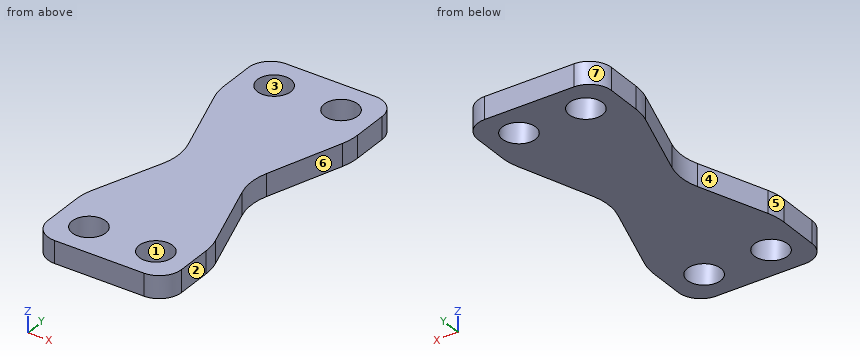
```python
from build123d import *

# Parameters (mm, degrees)
F0_R     = 1.5
F1_DEPTH = 2


with BuildPart() as f1:
    # F0 (on Top) → F1 (new body)
    with BuildSketch(Plane.XY):
        with BuildLine():
            ThreePointArc((-57.214044, -21.459296), (-56.628257, -22.87351), (-55.214044, -23.459296))
            Line((-55.214044, -23.459296), (-47.214044, -23.459296))
            ThreePointArc((-47.214044, -23.459296), (-45.79983, -22.87351), (-45.214044, -21.459296))
            Line((-45.214044, -21.459296), (-45.214044, -18.270684))
            ThreePointArc((-45.214044, -18.270684), (-45.278606, -17.469773), (-45.470627, -16.689545))
            Line((-45.470627, -16.689545), (-47.686997, -10.040435))
            ThreePointArc((-47.686997, -10.040435), (-47.943581, -8.459296), (-47.686997, -6.878157))
            Line((-47.686997, -6.878157), (-45.470627, -0.229047))
            ThreePointArc((-45.470627, -0.229047), (-45.278606, 0.551181), (-45.214044, 1.352092))
            Line((-45.214044, 1.352092), (-45.214044, 4.540704))
            ThreePointArc((-45.214044, 4.540704), (-45.79983, 5.954918), (-47.214044, 6.540704))
            Line((-47.214044, 6.540704), (-55.214044, 6.540704))
            ThreePointArc((-55.214044, 6.540704), (-56.628257, 5.954918), (-57.214044, 4.540704))
            Line((-57.214044, 4.540704), (-57.214044, 1.352092))
            ThreePointArc((-57.214044, 1.352092), (-57.149481, 0.551181), (-56.95746, -0.229047))
            Line((-56.95746, -0.229047), (-54.7577, -6.828327))
            ThreePointArc((-54.7577, -6.828327), (-54.501338, -8.456588), (-54.788344, -10.079728))
            Line((-54.788344, -10.079728), (-56.926816, -16.113589))
            ThreePointArc((-56.926816, -16.113589), (-57.141713, -16.936462), (-57.214044, -17.783851))
            Line((-57.214044, -17.783851), (-57.214044, -21.459296))
        make_face()
        with Locations((-54.214044, -20.459296)):
            Circle(F0_R, mode=Mode.SUBTRACT)
        with Locations((-48.214044, -20.459296)):
            Circle(F0_R, mode=Mode.SUBTRACT)
        with Locations((-54.214044, 3.540704)):
            Circle(F0_R, mode=Mode.SUBTRACT)
        with Locations((-48.214044, 3.540704)):
            Circle(F0_R, mode=Mode.SUBTRACT)
    extrude(amount=F1_DEPTH)


solid = f1.part
```
The model under review builds one solid part; all positions refer to its coordinate system, in mm. Face numbers are marked on the shaded views. A direction names the side the tool comes from. Give positions to 0.01 mm unless a question says otherwise; leave off trailing zeros. Write each loop counter-clockwise with the first axis right and the second up, starting at its lowest first coordinate (ties: lowest second). Pieces come first, ordered by that corner, then holes.
(1) Consider section B-B, the plane x = -46.25. Give the boundary of the cut face in (y, z), and give its area (3 significant figures).
(2) Consider section A-A, the plane x = -54. Give the boundary of the cut face in (y, z), and give its area (3 significant figures).
(3) The part is to be moulded in two halves that separate along X. For the marked faces 1, 2, 3 and 4, say which applies: released by +X, released by -X, zero draft, split by the parting line, or undercut.
(4) Consider section D-D, the plane x = -49. Give the boundary of the cut face in (y, z).
(5) Tool access review of the marked faces 5, 6 and 7: name each direction out of +Z, -Z, +X, -X, +Y, -Y from which nothing blocks a thin tool from reaching the whole face with its end or side.
(6) To check wall thickness, follow L1, parallel to X at y = 4, z = 1.45; L2, parallel to Y at x = -48.75, z = 0.65; L3, parallel to Y at x = -48.5, z = 1.35. State the ranges of each line that lie inside material, in increasing order.
(7) Consider section C-C, the plane z = 0.6. Give the boundary of the cut face in (x, y).
Returned:
1. outline: (-23.21, 0) - (-14.35, 0) - (-14.35, 2) - (-23.21, 2) - close; (-2.57, 0) - (6.29, 0) - (6.29, 2) - (-2.57, 2) - close
1. area: 35.4 mm2
2. outline: (-23.46, 0) - (-21.94, 0) - (-21.94, 2) - (-23.46, 2) - close; (-18.97, 0) - (2.06, 0) - (2.06, 2) - (-18.97, 2) - close; (5.03, 0) - (6.54, 0) - (6.54, 2) - (5.03, 2) - close
2. area: 48.1 mm2
3. face 1: undercut
3. face 2: released by +X
3. face 3: undercut
3. face 4: released by -X
4. outline: (-23.46, 0) - (-21.74, 0) - (-21.74, 2) - (-23.46, 2) - close; (-19.18, 0) - (2.26, 0) - (2.26, 2) - (-19.18, 2) - close; (4.82, 0) - (6.54, 0) - (6.54, 2) - (4.82, 2) - close
5. face 5: +Z, -Z, -X
5. face 6: +Z, -Z, +X
5. face 7: +Z, -Z, -X, +Y
6. L1: x = -57.21 to -55.64, -52.79 to -49.64, -46.79 to -45.21
6. L2: y = -23.46 to -21.86, -19.06 to 2.14, 4.94 to 6.54
6. L3: y = -23.46 to -21.93, -18.99 to 2.07, 5.01 to 6.54
7. outline: (-57.21, -21.46) arc R2 ccw to (-55.21, -23.46) - (-47.21, -23.46) arc R2 ccw to (-45.21, -21.46) - (-45.21, -18.27) arc R5 ccw to (-45.47, -16.69) - (-47.69, -10.04) arc R5 cw to (-47.69, -6.88) - (-45.47, -0.23) arc R5 ccw to (-45.21, 1.35) - (-45.21, 4.54) arc R2 ccw to (-47.21, 6.54) - (-55.21, 6.54) arc R2 ccw to (-57.21, 4.54) - (-57.21, 1.35) arc R5 ccw to (-56.96, -0.23) - (-54.76, -6.83) arc R5 cw to (-54.79, -10.08) - (-56.93, -16.11) arc R5 ccw to (-57.21, -17.78) - close; hole circle Ø3 at (-54.21, -20.46); hole circle Ø3 at (-54.21, 3.54); hole circle Ø3 at (-48.21, -20.46); hole circle Ø3 at (-48.21, 3.54)
